Geometry check sheet. Reference: the model listing, model coordinates, mm. A direction names the side the tool comes from. Coordinates: 2 decimals unless noted, no trailing zeros. Order: outer loops, then holes, each group sorted by start corner. A loop starts at its lowest first (then second) coordinate and runs counter-clockwise, first axis right, second up. Notation, with made-up numbers: (-33, -28.75) -> (0, -28.75) arc R29 ccw to (0, 1.25) -> close; hole circle Ø8 at (32, 56). An arc over 180 degrees is marked (long way). Answer as CSV lines item,"result". Start each with the question number.
from build123d import *

# Parameters (mm, degrees)
SKETCH_1_R          = 4
EXTRUDE_1_DEPTH     = 1.3
SKETCH_2_R          = 2
EXTRUDE_2_DEPTH     = 25
CUT_EXTRUDE_1_DEPTH = 1.2
FILLET_1_R          = 0.8


with BuildPart() as part:
    # 草图1 → 凸台-拉伸1 (new body)
    with BuildSketch(Plane.XY):
        Circle(SKETCH_1_R)
    extrude(amount=EXTRUDE_1_DEPTH)

    # 草图2 → 凸台-拉伸2 (add)
    with BuildSketch(Plane.XY.offset(1.3)):
        Circle(SKETCH_2_R)
    extrude(amount=EXTRUDE_2_DEPTH)

    # 草图3 → 切除-拉伸1 (cut)
    with BuildSketch(Plane(origin=(0, 0, 0), x_dir=(-1, 0, 0), z_dir=(0, 0, -1))):
        Polygon((-0.721687836, 1.25), (-1.443375673, 0), (-0.721687836, -1.25), (0.721687836, -1.25), (1.443375673, 0), (0.721687836, 1.25), align=None)
    extrude(amount=-CUT_EXTRUDE_1_DEPTH, mode=Mode.SUBTRACT)

    # 圆角1
    fillet_1_edges = [part.edges().sort_by_distance(p)[0] for p in [
        (-4, 0, 0),
    ]]
    fillet(fillet_1_edges, radius=FILLET_1_R)


solid = part.part
Q1. Go/stop test with flat-tipped pins: pin 1 Ø1.2 at (x, y) = (0.5, 0) entering from -Z; pin 2 Ø2 at (y, z) = (0.5, 8) entering from -X. Record where each tip stops, or that it passes through.
Q2. Thickness scan on L1, parallel to Z at x = 0.5, y = -2; L2, parallel to Z at x = -0.5, y = -0.75; L3, parallel to X at y = 1, z = 11.75. Record the ranges inside material, lowest first.
Q3. Sectioned sample at A-A, the plane x = 0. Record the cut outline in (y, z).
Q4. Release check for a two-part mould opening along X. For faces 1 (the cylindrical face through (-0.867, -3.905, 1.046)), 2 (the flat face through (1.4, -0.7, 0)), 3 (the flat face through (0, 1.25, 1)) record: released by +X, released by -X, zero draft, split by the parting line, or undercut.
Q5. Sectioned sample at B-B, the plane z = 5. Record the cut outline in (x, y).
Q6. Access from +Z, -Z, +X, -X, +Y, -Y to the whole of each face (thin tool, end or side, straight path). Record for faces 4 (the flat face through (1.088, -0.616, 0.592)), 5 (the flat face through (0, 0, 26.3)), 6 (the cylindrical face through (0, -2, 14)).
Geometry results:
1,pin 1,"stops at z = 1.2"
1,pin 2,"stops at x = -2"
2,L1,"z = 0 to 1.3"
2,L2,"z = 1.2 to 26.3"
2,L3,"x = -1.73 to 1.73"
3,outline,"(-4, 0.8) arc R0.8 ccw to (-3.2, 0) -> (-1.25, 0) -> (-1.25, 1.2) -> (1.25, 1.2) -> (1.25, 0) -> (3.2, 0) arc R0.8 ccw to (4, 0.8) -> (4, 1.3) -> (2, 1.3) -> (2, 26.3) -> (-2, 26.3) -> (-2, 1.3) -> (-4, 1.3) -> close"
4,face 1,"split by the parting line"
4,face 2,"zero draft"
4,face 3,"undercut"
5,outline,"circle Ø4 at (0, 0)"
6,face 4,"-Z"
6,face 5,"+Z, +X, -X, +Y, -Y"
6,face 6,"+Z"
